from build123d import *

# Parameters (mm, degrees)
SKETCH2_W           = 0.35
SKETCH2_H           = 1.25
CUT_EXTRUDE1_DEPTH  = 1
SKETCH3_W           = 1.5
SKETCH3_H           = 0.25
BOSS_EXTRUDE1_DEPTH = 0.25


with BuildPart() as part:
    # Sketch1 → Revolve1 (revolve)
    with BuildSketch(Plane(origin=(0, 0, 0), x_dir=(0, 0, -1), z_dir=(1, 0, 0))):
        Polygon((0, 5.75), (-5.75, 5.75), (-5.75, -2.25), (-5.5, -2.25), (-5.5, -5.75), (0, -5.75), align=None)
    revolve(axis=Axis((0, 5.75, 0), (0, -1, 0)))

    # Sketch2 → Cut-Extrude1 (cut)
    with BuildSketch(Plane.XZ.offset(5.75)):
        with Locations((0, -1.875)):
            Rectangle(SKETCH2_W, SKETCH2_H)
        with Locations((2.8, 1.875)):
            Rectangle(SKETCH2_W, SKETCH2_H)
        with Locations((0, 1.875)):
            Rectangle(SKETCH2_W, SKETCH2_H)
        with Locations((2.8, -1.875)):
            Rectangle(SKETCH2_W, SKETCH2_H)
        with Locations((-2.8, -1.875)):
            Rectangle(SKETCH2_W, SKETCH2_H)
        with Locations((-2.8, 1.875)):
            Rectangle(SKETCH2_W, SKETCH2_H)
        with BuildLine():
            ThreePointArc((5.334266585, 1.34), (3.994266585, 0), (5.334266585, -1.34))
            ThreePointArc((5.334266585, -1.34), (5.5, 0), (5.334266585, 1.34))
        make_face()
        with BuildLine():
            ThreePointArc((-5.334266585, 1.34), (-3.994266585, 0), (-5.334266585, -1.34))
            ThreePointArc((-5.334266585, -1.34), (-5.5, 0), (-5.334266585, 1.34))
        make_face()
    extrude(amount=-CUT_EXTRUDE1_DEPTH, mode=Mode.SUBTRACT)

    # Sketch3 → Boss-Extrude1 (add)
    with BuildSketch(Plane.XZ.offset(5.75)):
        Polygon((1.25, -0.125), (1.875, -0.125), (1.875, -0.75), (2.125, -0.75), (2.125, -0.125), (2.75, -0.125), (2.75, 0.125), (2.125, 0.125), (2.125, 0.75), (1.875, 0.75), (1.875, 0.125), (1.25, 0.125), align=None)
        with Locations((-2, 0)):
            Rectangle(SKETCH3_W, SKETCH3_H)
    extrude(amount=BOSS_EXTRUDE1_DEPTH)


solid = part.part
CAD build for the part. Positions are in the model's coordinates, mm. A direction names the side the tool comes from. Coordinates: 2 decimals unless noted, no trailing zeros. Loops run counter-clockwise (first coordinate to the right, second up) from the corner with the lowest first, then second, coordinate; pieces in that order, holes last. Notation, with made-up numbers: (-38.75, 49.5) -> (-26.75, 49.5) arc R22 ccw to (-26.75, 69.5) -> close; hole circle Ø4 at (6.5, 19.5). An arc over 180 degrees is marked (long way). One line per item, written item: value.
1. Pull direction X, two halves, no side cores. Call faces 4 (the face through (-3.995, -5.257, 0.029)), 5 (the face through (2, -6, 0)), 6 (the face through (-2.625, -5, 2)): pulls with the +X half, pulls with the -X half, needs draft (parallel to the pull), parting line crosses it, or undercut.
Answers:
face 4: pulls with the -X half
face 5: needs draft
face 6: undercut
2. Slice it at C-C on y = 4. Write the cut outline in (x, z).
Answers:
outline: circle Ø11.5 at (0, 0)
3. Flat gauge pins, fed straight in: P1, Ø0.5, axis at y = -5.5, z = -1.5, coming from the -X side; P2, Ø0.5, axis at y = -5, z = 1.5, coming from the +X side; P3, Ø1.5, axis at y = 0, z = -1.5, coming from the +X side. Where does each tip first touch, or does it go through?
Answers:
P1: stops at x = -5.33
P2: stops at x = 5.33
P3: stops at x = 5.7
4. Slice it at A-A on x = 0. Write the cut outline in (y, z), and give its area (3 significant figures).
Answers:
outline: (-5.75, -5.5) -> (-2.25, -5.5) -> (-2.25, -5.75) -> (5.75, -5.75) -> (5.75, 5.75) -> (-2.25, 5.75) -> (-2.25, 5.5) -> (-5.75, 5.5) -> (-5.75, 2.5) -> (-4.75, 2.5) -> (-4.75, 1.25) -> (-5.75, 1.25) -> (-5.75, -1.25) -> (-4.75, -1.25) -> (-4.75, -2.5) -> (-5.75, -2.5) -> close
area: 128 mm^2
5. Slice it at D-D on z = 4.5. Write the cut outline in (x, y), and give its area (3 significant figures).
Answers:
outline: (-3.58, -2.25) -> (-3.16, -2.25) -> (-3.16, -5.75) -> (3.16, -5.75) -> (3.16, -2.25) -> (3.58, -2.25) -> (3.58, 5.75) -> (-3.58, 5.75) -> close
area: 79.4 mm^2
6. Which spindle directions (+Z, -Z, +X, -X, +Y, -Y) get a long thin tool onto all of the face, cutting with end or side? Do faces 1 (the face through (5, -4.75, 0)), 2 (the face through (-5, -4.75, 0)), 3 (the face through (2.975, -5, -2)). Say none if no direction does.
Answers:
face 1: +X, -Y
face 2: -X, -Y
face 3: -Y
7. Drill centre lines: line 1 (Z direction, x = 0, y = -5.25); line 2 (Y direction, x = -1, z = 1.25); line 3 (Z direction, x = 0, y = -3.25). Where is each one in solid material? Low to high. Write a range as [from, to].
Answers:
line 1: z = [-5.5, -2.5], [-1.25, 1.25], [2.5, 5.5]
line 2: y = [-5.75, 5.75]
line 3: z = [-5.5, 5.5]
8. Slice it at B-B on z = -3.25. Write the cut outline in (x, y), and give its area (3 significant figures).
Answers:
outline: (-4.74, -2.25) -> (-4.44, -2.25) -> (-4.44, -5.75) -> (4.44, -5.75) -> (4.44, -2.25) -> (4.74, -2.25) -> (4.74, 5.75) -> (-4.74, 5.75) -> close
area: 107 mm^2
